The figure shows three views and two pictorial views of one solid part (mm, origin at its lowest corner). Answer the questions. Coordinates: 2 decimals unless noted, no trailing zeros. Loops run counter-clockwise (first coordinate to the right, second up) from the corner with the lowest first, then second, coordinate; pieces in that order, holes last. Notation, with made-up numbers: (13, -1.5) -> (69, -1.5) arc R16 ccw to (69, 6.5) -> close; hole circle Ø3 at (-7.75, 11). An arc over 180 degrees is marked (long way). Answer as a JSON object with one key per item and string values. Group by question number.
1) Consider probe 1 along Z at (x, y) = (19, 43). Determine where the line is inside the solid, lowest interval first. Write a range as [from, to].
2) Section A-A, the plane x = 41.5 is taken. Give the vertices of the cut face in (y, z), plus the area to 4 significant figures.
3) Flat-ended cylindrical pins translate along their axes: P1, Ø10, axis at x = 45, y = 9.5, coming from the -Z side; P2, Ø10.5, axis at y = 45.5, z = 31.5, coming from the -X side; P3, Ø10.5, axis at x = 35, z = 2063, coming from the +Y side. Find the tip coordinate at first contact, or state that the pin passes through.
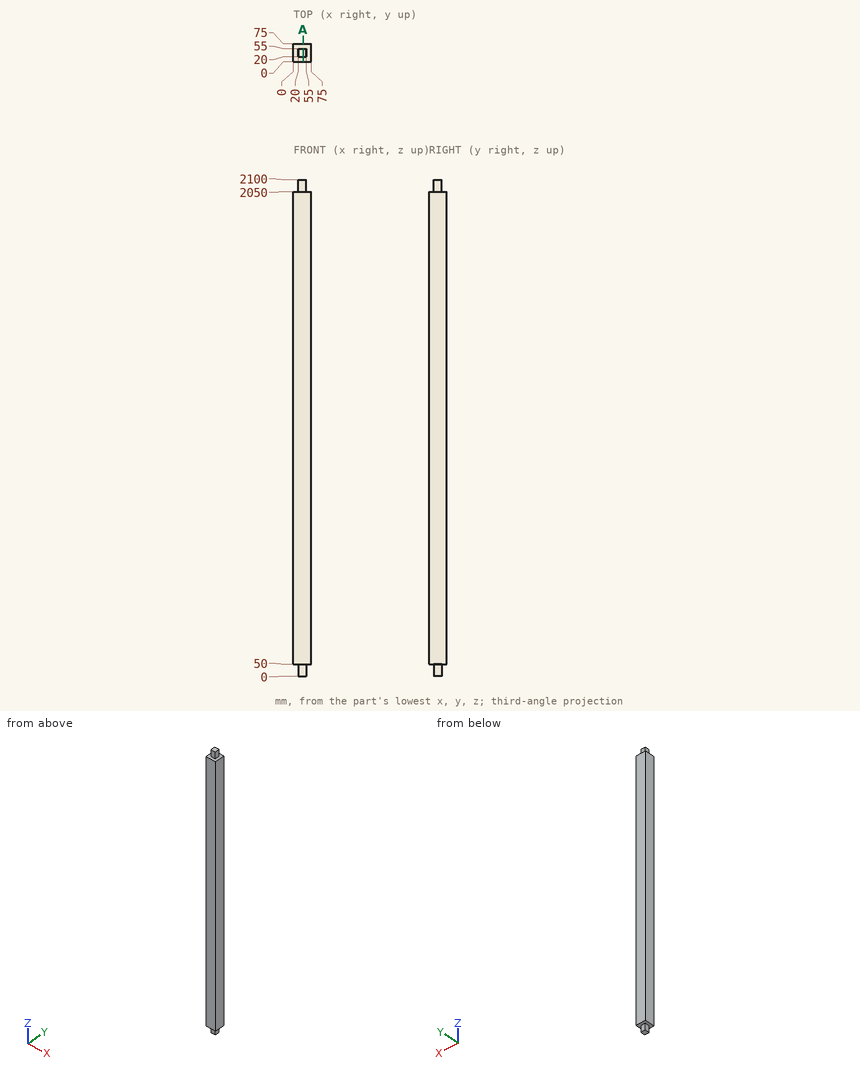
Determined:
{
 "1": {"probe 1": "[50, 2050]"},
 "2": {"outline": "(0, 50) -> (20, 50) -> (20, 0) -> (55, 0) -> (55, 50) -> (75, 50) -> (75, 2050) -> (55, 2050) -> (55, 2100) -> (20, 2100) -> (20, 2050) -> (0, 2050) -> close", "area": "153,500 mm²"},
 "3": {"P1": "z = 50", "P2": "x = 20", "P3": "y = 55"}
}
